For this review, take the finished solid that the model builds, in its own axes (mm). Coordinates: 2 decimals unless noted, no trailing zeros. Loops run counter-clockwise (first coordinate to the right, second up) from the corner with the lowest first, then second, coordinate; pieces in that order, holes last.
1. Take a section at D-D, the plane y = 9.5. State the section outline as (x, z) points (1 decimal).
2. To check wall thickness, follow probe 1 along X at (y, z) = (10.25, -1); probe 2 along X at (y, z) = (6, 2); probe 3 along Z at (x, y) = (8.5, 5). State the ranges of each line that lie inside material, in increasing order.
3. Clearance check with flat-ended pins moving along their axes: P1, Ø5.5, axis at x = -3.5, z = 1.5, coming from the -Y side; P2, Ø1.5, axis at x = 2.5, y = 7.5, coming from the -Z side; P3, Ø1.5, axis at y = 4, z = 2, coming from the -X side. State where each tip first meets the part, or that it passes through.
4. Take a section at C-C, the plane y = 2. State the section outline as (x, z) points (1 decimal).
5. Mouldability with a two-part tool opening along X and no side actions: class faces 1 (the face through (-0.628, 6.432, 14.274)), 2 (the face through (2.435, 2.475, -0.767)), 3 (the face through (-9.4, 0, 2.9)), 4 (the face through (2, 0.762, 2)) as pulls with the +X half, pulls with the -X half, needs draft (parallel to the pull), parting line crosses it, or undercut.
```python
from build123d import *

# Parameters (mm, degrees)
FILLET1_R               = 0.508
F_1_4_20_TAPPED_HOLE1_D = 5.1054


with BuildPart() as part:
    # Sketch1 → Revolve1 (revolve)
    with BuildSketch(Plane.XY, mode=Mode.PRIVATE) as revolve1_sk:
        Polygon((0, 0.762), (8.763, 0.762), (9.525, 0), (14.2875, 0), (14.2875, 12.7), (11.1125, 12.7), (0, 1.5875), align=None)
    revolve(revolve1_sk.sketch.rotate(Axis((0, 0, 0), (0, 1, 0)), 90), axis=Axis((0, 0, 0), (0, 1, 0)))  # turned: the seam where the file's is

    # Fillet1
    fillet1_edges = [part.edges().sort_by_distance(p)[0] for p in [
        (0, 0, 14.2875),
        (0, 12.7, 14.2875),
        (0, 12.7, 11.1125),
    ]]
    fillet(fillet1_edges, radius=FILLET1_R)

    # 1_4-20 Tapped Hole1 (through all)
    with Locations(Plane(origin=(0, 0.762, 0), x_dir=(-1, 0, 0), z_dir=(0, -1, 0))):
        with Locations((0, 0)):
            Hole(F_1_4_20_TAPPED_HOLE1_D / 2)


solid = part.part
```
Results list:
1. outline: circle Ø28.6 at (0, 0); hole circle Ø15.8 at (0, 0)
2. probe 1: x = -14.25 to -8.6, 8.6 to 14.25
2. probe 2: x = -14.15 to -3.93, 3.93 to 14.15
2. probe 3: z = -11.48 to 11.48
3. P1: stops at y = 0.76
3. P2: stops at z = -14.18
3. P3: stops at x = -14.23
4. outline: circle Ø28.6 at (0, 0); hole circle Ø5.1 at (0, 0)
5. face 1: parting line crosses it
5. face 2: undercut
5. face 3: needs draft
5. face 4: undercut
